Here's how the part is built. I have some questions about the finished solid (model axes, mm). Coordinates: 2 decimals unless noted, no trailing zeros. Loops run counter-clockwise (first coordinate to the right, second up) from the corner with the lowest first, then second, coordinate; pieces in that order, holes last.
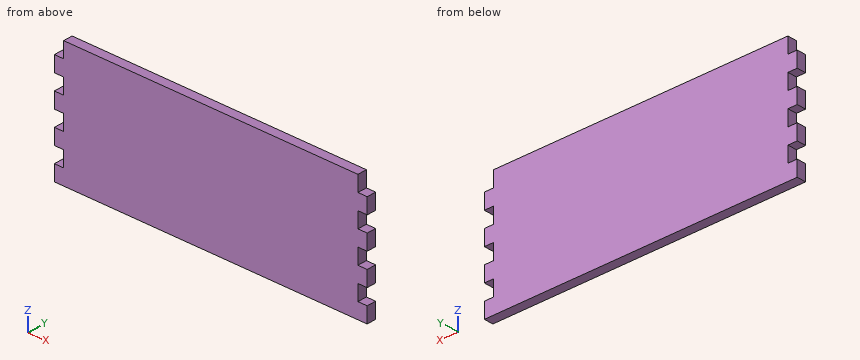
```python
from build123d import *

# Parameters (mm, degrees)
F0_W     = 95
F0_H     = 40
F1_DEPTH = 3
F2_W     = 3
F2_H     = 5
F3_DEPTH = 3


# Not quite as in the source:
# - a feature names something its author has since deleted; it is built from what else it names


with BuildPart() as f1:
    # F0 (on Front) → F1 (new body)
    with BuildSketch(Plane.XZ):
        Rectangle(F0_W, F0_H)
    extrude(amount=F1_DEPTH)

    # F2 (on face) → F3 (join)
    with BuildSketch(Plane.XZ.offset(3)):
        with Locations((-49, -17.5)):
            Rectangle(F2_W, F2_H)
        with Locations((-49, -7.5)):
            Rectangle(F2_W, F2_H)
        with Locations((-49, 2.5)):
            Rectangle(F2_W, F2_H)
        with Locations((-49, 12.5)):
            Rectangle(F2_W, F2_H)
        with Locations((49, -7.5)):
            Rectangle(F2_W, F2_H)
        with Locations((49, -17.5)):
            Rectangle(F2_W, F2_H)
        with Locations((49, 12.5)):
            Rectangle(F2_W, F2_H)
        with Locations((49, 2.5)):
            Rectangle(F2_W, F2_H)
    extrude(amount=-F3_DEPTH)


solid = f1.part
```
1. For pin 1 (1.5 mm diameter, centred on x = 49, y = -1.5, fed in from +Z); pin 2 (1.5 mm diameter, centred on y = -1, z = -13, fed in from +X); pin 3 (1.5 mm diameter, centred on y = -2, z = -13.5, fed in from -X), each with a flat end and sliding along its axis, tell me the tip position at first contact or that it passes through.
2. I need wall thicknesses on line 1 along X through (y, z) = (-1.25, 16). Which ranges of the line are inside material? Lowest first, please.
3. I want a section at B-B (z = 17.5). Please give me the cut outline in (x, y), then the cut area to 3 significant figures.
Response values:
1. pin 1: stops at z = 15
1. pin 2: stops at x = 47.5
1. pin 3: stops at x = -47.5
2. line 1: x = -47.5 to 47.5
3. outline: (-47.5, -3) - (47.5, -3) - (47.5, 0) - (-47.5, 0) - close
3. area: 285 mm2
